Geometry check sheet. Reference: the model listing, model coordinates, mm. Face numbers are marked on the shaded views. A direction names the side the tool comes from. Round coordinates to 2 decimals unless told otherwise and drop trailing zeros. Loops run counter-clockwise (first coordinate to the right, second up) from the corner with the lowest first, then second, coordinate; pieces in that order, holes last. Notation, with made-up numbers: (-4.5, -28.75) - (26.5, -28.75) arc R11 ccw to (26.5, -23.75) - close; hole circle Ø11 at (22.25, 57). An arc over 180 degrees is marked (long way). Write item = value, one per line.
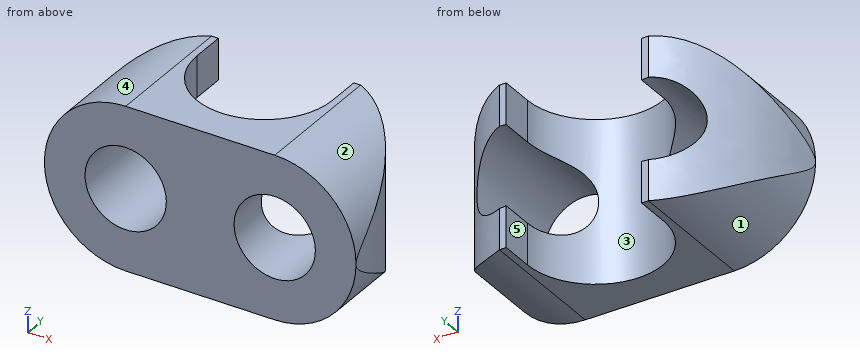
```python
from build123d import *

# Parameters (mm, degrees)
ESBO_O1_R                = 3
RESSALTO_EXTRUS_O1_DEPTH = 10
CORTE_EXTRUS_O1_DEPTH    = 20.397164741
CORTE_EXTRUS_O2_DEPTH    = 20.397164855


with BuildPart() as part:
    # Esboço1 → Ressalto-extrusão1 (new body)
    with BuildSketch(Plane(origin=(0, 0, 0), x_dir=(1, 0, 0), z_dir=(0, 1, 0))):
        with BuildLine():
            Line((-5.5, -6), (5.5, -6))
            ThreePointArc((5.5, -6), (11.5, 0), (5.5, 6))
            Line((5.5, 6), (-5.5, 6))
            ThreePointArc((-5.5, 6), (-11.5, 0), (-5.5, -6))
        make_face()
        with Locations(Location((-5.5, 0, 0), (0, 0, 270))):
            Circle(ESBO_O1_R, mode=Mode.SUBTRACT)
        with Locations(Location((5.5, 0, 0), (0, 0, 270))):
            Circle(ESBO_O1_R, mode=Mode.SUBTRACT)
    extrude(amount=RESSALTO_EXTRUS_O1_DEPTH)

    # Esboço2 → Corte-extrusão1 (cut, through all)
    with BuildSketch(Plane.XY.offset(6)):
        with BuildLine():
            Line((-5, 7.5), (-5, 10))
            Line((-5, 10), (5, 10))
            Line((5, 10), (5, 7.5))
            ThreePointArc((5, 7.5), (0, 2.5), (-5, 7.5))
        make_face()
    extrude(amount=-CORTE_EXTRUS_O1_DEPTH, mode=Mode.SUBTRACT)

    # Esboço3 → Corte-extrusão2 (cut, through all)
    with BuildSketch(Plane.XY.offset(6)):
        with BuildLine():
            Line((-11.5, 10), (-11.5, 0))
            add(Edge.make_bspline(
                [(-11.5, 0), (-10.890573495, 7.573019438), (-5.5, 10)],
                knots=[0, 0, 0, 0.339761367, 0.339761367, 0.339761367], degree=2))
            Line((-5.5, 10), (-11.5, 10))
        make_face()
        with BuildLine():
            Line((11.5, 10), (5.5, 10))
            add(Edge.make_bspline(
                [(5.5, 10), (10.890573495, 7.573019438), (11.5, 0)],
                knots=[0.660238633, 0.660238633, 0.660238633, 1, 1, 1], degree=2))
            Line((11.5, 0), (11.5, 10))
        make_face()
    extrude(amount=-CORTE_EXTRUS_O2_DEPTH, mode=Mode.SUBTRACT)


solid = part.part
```
(1) Gauge pin test, flat ends, axial feed: pin 1 (2 mm diameter, centred on y = 3, z = -0.5, fed in from -X); pin 2 (1.5 mm diameter, centred on y = 4.5, z = -2, fed in from -X); pin 3 (1.2 mm diameter, centred on y = 8, z = -4, fed in from +X); pin 4 (5.5 mm diameter, centred on x = 5.5, z = 0, fed in from -Y). Record the tip position at first contact, or that the pin passes through.
Answers follow:
pin_1 = -11.24
pin_2 = -10.81
pin_3 = 8.92
pin_4 = through
(2) Mould release check, pull along X, two halves, no side actions. Record for the marked faces 1, 2 and 3: pulls with the +X half, pulls with the -X half, needs draft (parallel to the pull), parting line crosses it, or undercut.
Answers follow:
face_1 = pulls with the -X half
face_2 = pulls with the +X half
face_3 = undercut
(3) Set-up check for the marked faces 4 and 5: record each of +Z, -Z, +X, -X, +Y, -Y from which the full face is reachable in a straight line by a thin tool's end or side.
Answers follow:
face_4 = +Z, -X, +Y, -Y
face_5 = +Z, -Z, +Y
(4) Section check A-A (y = 8.25). State how many separate pieces and enclosed holes the cut face has, then the cut area to 3 significant figures.
Answers follow:
separate_pieces = 4
enclosed_holes = 0
area = 40.2 mm²
(5) Section check B-B (x = 0). Enter the section's corners in (y, z), then the cut area to 3 significant figures.
Answers follow:
outline = (0, -6) - (2.5, -6) - (2.5, 6) - (0, 6) - close
area = 30.0 mm²
(6) Scan lines: L1, parallel to X at y = 0.5, z = -1.25; L2, parallel to X at y = 3, z = 2.75; L3, parallel to X at y = 0.75, z = -1.75. Record each from-to range of solid material in increasing order. Write a range as [from, to].
Answers follow:
L1 = [-11.37, -8.23], [-2.77, 2.77], [8.23, 11.37]
L2 = [-10.83, -6.7], [-4.3, -2.18], [2.18, 4.3], [6.7, 10.83]
L3 = [-11.24, -7.94], [-3.06, 3.06], [7.94, 11.24]
